Could you check a few things on this drawing? It's one solid part, dimensions in mm from its lowest x, y, z. A direction names the side the tool comes from. Give positions to 0.01 mm unless a question says otherwise; leave off trailing zeros. Loops run counter-clockwise (first coordinate to the right, second up) from the corner with the lowest first, then second, coordinate; pieces in that order, holes last.
1. Imagine slicing it at A-A (y = 12). List the corners of the cut face in (x, z) for me, plus the area to 3 significant figures.
2. Imagine slicing it at B-B (z = 23). List the corners of the cut face in (x, y) for me.
3. For the marked faces 4 and 5, which set-ups out of +Z, -Z, +X, -X, +Y, -Y let a thin tool reach every point of the face, with its end or its side?
4. Imagine slicing it at C-C (z = 10.5). List the corners of the cut face in (x, y) for me.
5. For P1, Ø7, axis at x = 14.5, y = 11, coming from the -Z side; P2, Ø8, axis at y = 21, z = 13, coming from the +X side; P3, Ø10, axis at x = 11.5, z = 47, coming from the -Y side, each with a flat end and sliding along its axis, tell me the tip position at first contact or that it passes through.
6. Thinking about a two-plate mould opening in Y: for the marked faces 1, 2 and 3, which applies, +Y half, -Y half, draft (parallel to the pull), parting line (faces both ways), or undercut?
7. I need wall thicknesses on line 1 along Z through (x, y) = (11, 9.25); line 2 along Z through (x, y) = (7.25, 8.25); line 3 along X through (y, z) = (11.75, 47) (1 decimal). Which ranges of each line are inside material? Lowest first, please.
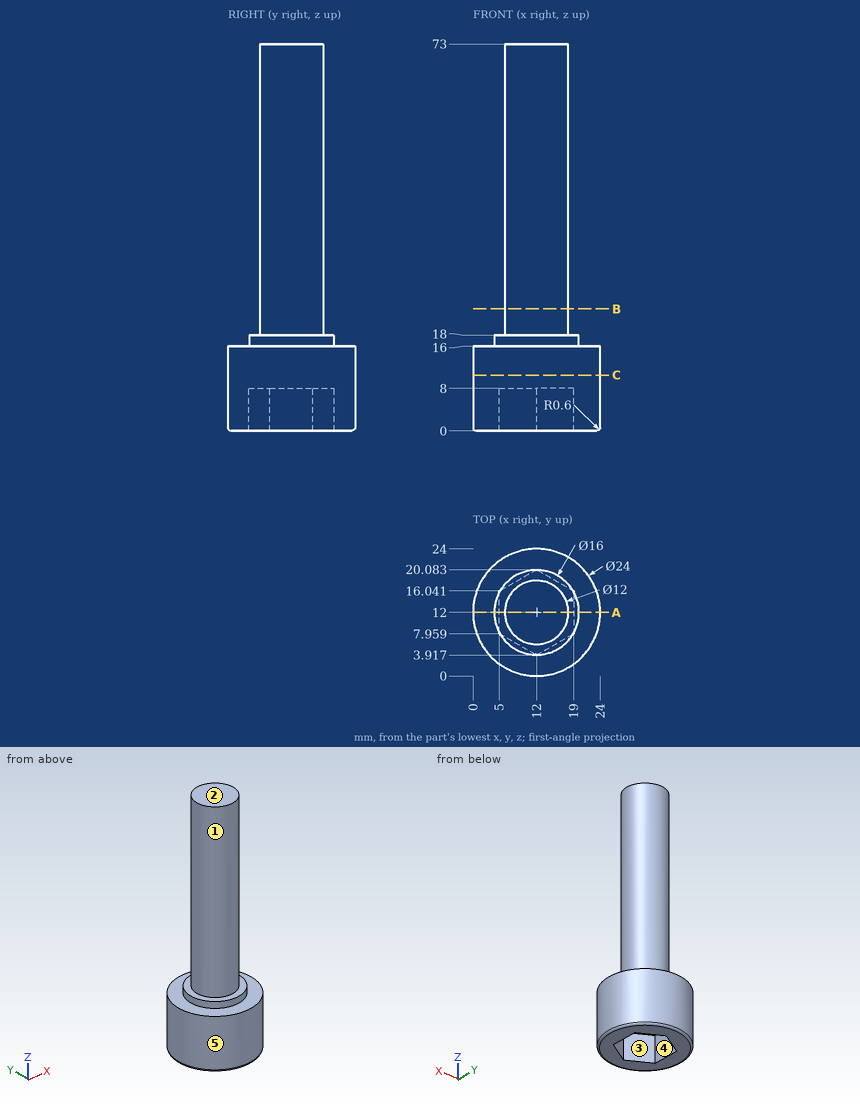
Derived:
1. outline: (0, 0.6) arc R0.6 ccw to (0.6, 0) - (5, 0) - (5, 8) - (19, 8) - (19, 0) - (23.4, 0) arc R0.6 ccw to (24, 0.6) - (24, 16) - (20, 16) - (20, 18) - (18, 18) - (18, 73) - (6, 73) - (6, 18) - (4, 18) - (4, 16) - (0, 16) - close
1. area: 964 mm2
2. outline: circle Ø12 at (12, 12)
3. face 4: -Z
3. face 5: +Z, -Z
4. outline: circle Ø24 at (12, 12)
5. P1: stops at z = 8
5. P2: stops at x = 22.91
5. P3: stops at y = 6
6. face 1: parting line
6. face 2: draft
6. face 3: undercut
7. line 1: z = 8 to 73
7. line 2: z = 8 to 18
7. line 3: x = 6 to 18
